Input: part model. Units: mm. Frame: model coordinates. Round coordinates to 2 decimals unless told otherwise and drop trailing zeros. Write each loop counter-clockwise with the first axis right and the second up, starting at its lowest first coordinate (ties: lowest second). Pieces come first, ordered by that corner, then holes. Notation, with made-up numbers: (30.5, 87) -> (87.5, 87) arc R14 ccw to (87.5, 91) -> close; hole circle Ø6 at (-29, -23.5). An arc over 180 degrees is marked (long way). Write item = value, one per line. Start each with the question number.
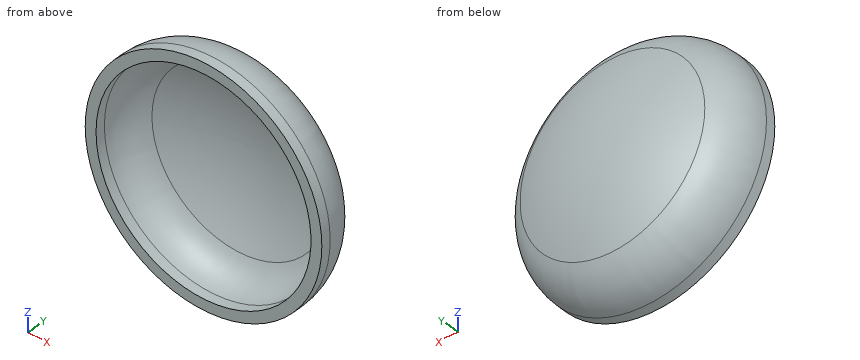
Autodesk Inventor part; units mm, degrees
ref_plane "YZ Plane" through (0, 0, 0) normal (1, 0, 0) x (0, 1, 0)
ref_plane "XZ Plane" through (0, 0, 0) normal (0, 1, 0) x (-1, 0, 0)
ref_plane "XY Plane" through (0, 0, 0) normal (0, 0, 1) x (1, 0, 0)
sketch "Sketch1" plane through (0, 0, 0) normal (0, 0, 1) x (1, 0, 0)
  arc A0 (0, 81.5958) -> (-112.6403, 54.6826) centre (0, -167.5782) ccw
  arc A1 (-112.6403, 54.6826) -> (-138.43, 12.7) centre (-91.3638, 12.7) ccw
  line L0 (-138.43, 12.7) -> (-138.43, 0)
  line L1 (-138.43, 0) -> (-152.4, 0)
  line L2 (-152.4, 0) -> (-152.4, 12.7)
  line L3 (0, 95.5658) -> (0, 81.5958)
  line L4 (0, -221.6084) -> (0, 156.6029)
  line L5 (-182.0818, 12.7) -> (-119.4588, 12.7) construction
  line L6 (-218.4982, 0) -> (36.4164, 0)
  arc A2 (-118.9555, 67.1437) -> (-152.4, 12.7) centre (-91.3638, 12.7) ccw
  arc A3 (0, 95.5658) -> (-118.9555, 67.1437) centre (0, -167.5782) ccw
  point P0 (-145.415, 0)
  dimension "Inner_D" = 138.43
  dimension "Thickness" = 13.97
  dimension "Skirt_Length" = 12.7
  dimension "Knuckle" = 47.0662
  dimension "Crown" = 249.174
  dimension "Thickness_Top" = 13.97
  dimension "Outside_Knuckle" = 61.0362
revolve "Revolution2" add sketch "Sketch1" angle 360 about axis through (0, -10, 0) along (0, 1, 0) contours A0 A1 L0 L1 L2 A2 A3 L3
equation "\"Thickness\" = Outlet_Cap_Wall_Thickness"
equation "\"Knuckle\" = Outlet_Cap_Knuckle_Radius"
properties part number "Fuel Cap Outlet"
1. Section A-A (y = 35.5). Output: boundary loops of the cut face in (x, z).
2. Pin query (flat end, axial travel): P1, Ø10, axis at y = 28.5, z = 111, coming from the +X side; P2, Ø4, axis at x = -29, z = 32, coming from the -Y side; P3, Ø1, axis at x = 42.5, y = 12.5, coming from the -Z side. Return the tip coordinate at first contact, or that it passes through.
3. Line query: line 1 along Z through (x, y) = (0, 9); line 2 along Z through (x, y) = (115.5, 21); line 3 along X through (y, z) = (7, 47). Output: solid intervals per line, ascending.
Check sheet entries:
q1.outline = circle Ø295.96 at (0, 0); hole circle Ø265.08 at (0, 0)
q2.P1 = 106.89
q2.P2 = 77.46
q2.P3 = -146.5
q3.line_1 = -152.4 to -138.43, 138.43 to 152.4
q3.line_2 = -98.55 to -74.96, 74.96 to 98.55
q3.line_3 = -144.97 to -130.21, 130.21 to 144.97
